CAD build for the part. Positions are in the model's coordinates, mm. Coordinates: 2 decimals unless noted, no trailing zeros. Loops run counter-clockwise (first coordinate to the right, second up) from the corner with the lowest first, then second, coordinate; pieces in that order, holes last. Notation, with made-up numbers: (36, 50) -> (80, 50) arc R15 cw to (80, 73) -> close; hole circle Ø9 at (-20, 72). An arc over 180 degrees is marked (long way). Write each question's results on one line, items separated by ' | '.
Autodesk Inventor part; units mm, degrees
ref_plane "Work Plane4" through (0, 0, -155) normal (0, 0, -1) x (-1, 0, 0)
ref_plane "Work Plane6" through (10, 10, -315) normal (0, -1, 0) x (-1, 0, 0)
ref_plane "YZ Plane" through (0, 0, 0) normal (1, 0, 0) x (0, 1, 0)
sketch "Sketch3" plane through (0, 0, 0) normal (0, 0, 1) x (1, 0, 0)
  circle A0 centre (0, 0) radius 4
  dimension "d11" = 8
extrude "Extrusion5" add sketch "Sketch3" against normal blind 310
sketch "Sketch4" plane through (0, 0, 0) normal (0, 0, 1) x (1, 0, 0)
  line L0 (-10, 10) -> (10, 10)
  line L1 (10, 10) -> (10, -10)
  line L2 (10, -10) -> (-10, -10)
  line L3 (-10, -10) -> (-10, 10)
  line L4 (-10, 10) -> (10, -10) construction
  line L5 (10, 10) -> (-10, -10) construction
  point P0 (0, 0)
  dimension "d17" = 20
  dimension "d18" = 20
extrude "Extrusion6" add sketch "Sketch4" along normal blind 5
ref_plane "Work Plane4" through (0, 0, -155) normal (0, 0, -1) x (-1, 0, 0)
mirror "Mirror1" about plane through (0, 0, -155) normal (0, 0, -1) of "Extrusion6"
ref_plane "Work Plane6" through (10, 10, -315) normal (0, -1, 0) x (-1, 0, 0)
ref_plane "Work Plane5" through (10, -10, -203.19) normal (0, 0, -1) x (-1, 0, 0)
sketch "Sketch5" plane through (10, 10, -315) normal (0, -1, 0) x (-1, 0, 0)
  line L0 (-4, -111.81) -> (24, -111.81) construction
  line L1 (14, -5) -> (6, -5) construction
  line L2 (6, -315) -> (14, -315) construction
  line L3 (0, -5) -> (20, -5) construction
  line L4 (10, -5) -> (10, -315) construction
  line L5 (6, -315) -> (6, -5) construction
  point P0 (10, -111.81)
hole "Hole1" at (0, 10, -203.19) direction (0, -1, 0) diameter 3.688 end through all
properties part number "rear axle" material "Steel, Mild"
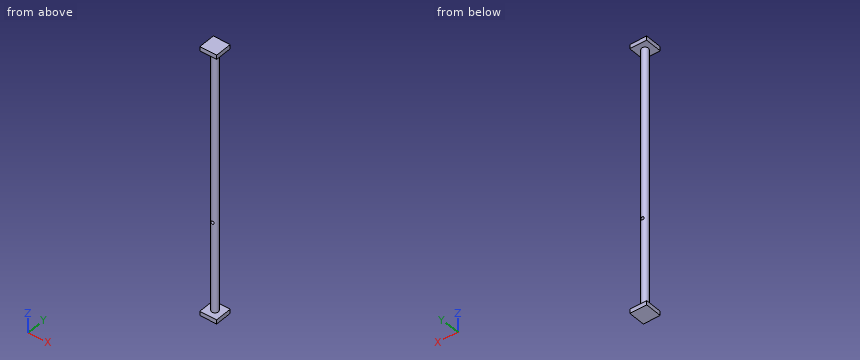
Q1. Drop flat-ended pins along their axis: pin 1 (8 mm diameter, centred on x = 4, z = -34.5, fed in from +Y); pin 2 (3 mm diameter, centred on x = 3.5, z = -34.5, fed in from +Y); pin 3 (1.5 mm diameter, centred on y = 2.5, z = -253.5, fed in from +X). Give the stop position or say it passes through.
Results are:
pin 1: y = 4 | pin 2: y = 3.46 | pin 3: x = 3.6
Q2. Wall check: L1, parallel to Z at x = -6.75, y = -7.5; L2, parallel to Z at x = 0, y = -1; L3, parallel to Y at x = -0.5, z = -19.5. Give the ranges that are in metal, low to high. Write a range as from..to.
Results are:
L1: -315..-310, 0..5 | L2: -315..-205.03, -201.35..5 | L3: -3.97..3.97
Q3. Cut at A-A on x = -6.75. Write the cut outline in (y, z).
Results are:
outline: (-10, -315) -> (10, -315) -> (10, -310) -> (-10, -310) -> close; (-10, 0) -> (10, 0) -> (10, 5) -> (-10, 5) -> close
Q4. Cut at C-C on z = -51. Write the cut outline in (x, y).
Results are:
outline: circle Ø8 at (0, 0)
Q5. Cut at B-B on y = 0. Write the cut outline in (x, z).
Results are:
outline: (-10, -315) -> (10, -315) -> (10, -310) -> (4, -310) -> (4, 0) -> (10, 0) -> (10, 5) -> (-10, 5) -> (-10, 0) -> (-4, 0) -> (-4, -310) -> (-10, -310) -> close; hole circle Ø3.69 at (0, -203.19)
